Design review of the part built by this model. Coordinates are the model's own, in mm. Coordinates: 2 decimals unless noted, no trailing zeros. Loops run counter-clockwise (first coordinate to the right, second up) from the corner with the lowest first, then second, coordinate; pieces in that order, holes last. Notation, with made-up numbers: (80.5, 84.25) -> (100.5, 84.25) arc R30 ccw to (100.5, 116.25) -> close; hole circle Ø5 at (-21, 44). An arc over 180 degrees is marked (long way). Use one line per item in the form item = value. Start each with the question number.
1. Consider section A-A (z = -27.5). State the section outline as (x, y) points, then the cut area to 3 significant figures.
2. Consider section C-C (x = 1.1). State the section outline as (y, z) points.
3. Consider section B-B (y = -17). State the section outline as (x, z) points.
4. For pin 1 (5.5 mm diameter, centred on y = 17, z = 27.5, fed in from +X); pin 2 (3 mm diameter, centred on y = -17, z = 27.5, fed in from -X), all flat-tipped, find the tip position at first contact; note any pin that passes through.
5. Wall thickness on line 1 (Y direction, x = 2.7, z = 27.5); line 2 (Y direction, x = 0.45, z = -27.5); line 3 (Z direction, x = 2.25, y = 18): over which ranges is each line inside the solid? List them lowest first. Write a range as from..to.
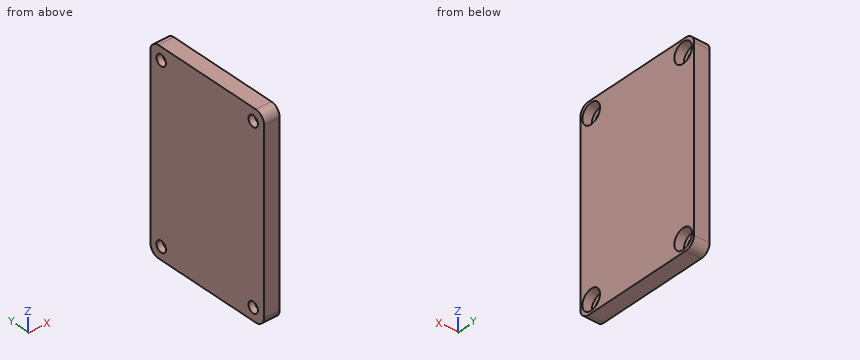
from build123d import *

# Parameters (mm, degrees)
BOSS_EXTRUDE1_DEPTH = 5
SKETCH2_R           = 1.75
CUT_EXTRUDE1_DEPTH  = 39.187039686
SKETCH3_R           = 3.25
CUT_EXTRUDE2_DEPTH  = 3


with BuildPart() as part:
    # Sketch1 → Boss-Extrude1 (new body)
    with BuildSketch(Plane.YZ):
        with BuildLine():
            Line((-18, -31.5), (18, -31.5))
            ThreePointArc((18, -31.5), (20.121320344, -30.621320344), (21, -28.5))
            Line((21, -28.5), (21, 28.5))
            ThreePointArc((21, 28.5), (20.121320344, 30.621320344), (18, 31.5))
            Line((18, 31.5), (-18, 31.5))
            ThreePointArc((-18, 31.5), (-20.121320344, 30.621320344), (-21, 28.5))
            Line((-21, 28.5), (-21, -28.5))
            ThreePointArc((-21, -28.5), (-20.121320344, -30.621320344), (-18, -31.5))
        make_face()
    extrude(amount=BOSS_EXTRUDE1_DEPTH)

    # Sketch2 → Cut-Extrude1 (cut, through all)
    with BuildSketch(Plane.YZ.offset(5)):
        with Locations(Location((-17, 27.5, 0), (0, 0, 270))):
            Circle(SKETCH2_R)
        with Locations(Location((17, 27.5, 0), (0, 0, 270))):
            Circle(SKETCH2_R)
        with Locations(Location((17, -27.5, 0), (0, 0, 270))):
            Circle(SKETCH2_R)
        with Locations(Location((-17, -27.5, 0), (0, 0, 270))):
            Circle(SKETCH2_R)
    extrude(amount=-CUT_EXTRUDE1_DEPTH, mode=Mode.SUBTRACT)

    # Sketch3 → Cut-Extrude2 (cut)
    with BuildSketch(Plane.YZ.offset(5)):
        with Locations(Location((17, 27.5, 0), (0, 0, 270))):
            Circle(SKETCH3_R)
        with Locations(Location((-17, 27.5, 0), (0, 0, 270))):
            Circle(SKETCH3_R)
        with Locations(Location((17, -27.5, 0), (0, 0, 270))):
            Circle(SKETCH3_R)
        with Locations(Location((-17, -27.5, 0), (0, 0, 270))):
            Circle(SKETCH3_R)
    extrude(amount=-CUT_EXTRUDE2_DEPTH, mode=Mode.SUBTRACT)


solid = part.part
Geometry check:
q1.outline = (0, -21) -> (5, -21) -> (5, -20.25) -> (2, -20.25) -> (2, -18.75) -> (0, -18.75) -> close; (0, -15.25) -> (2, -15.25) -> (2, -13.75) -> (5, -13.75) -> (5, 13.75) -> (2, 13.75) -> (2, 15.25) -> (0, 15.25) -> close; (0, 18.75) -> (2, 18.75) -> (2, 20.25) -> (5, 20.25) -> (5, 21) -> (0, 21) -> close
q1.area = 157 mm²
q2.outline = (-21, -28.5) arc R3 ccw to (-18, -31.5) -> (18, -31.5) arc R3 ccw to (21, -28.5) -> (21, 28.5) arc R3 ccw to (18, 31.5) -> (-18, 31.5) arc R3 ccw to (-21, 28.5) -> close; hole circle Ø3.5 at (-17, -27.5); hole circle Ø3.5 at (-17, 27.5); hole circle Ø3.5 at (17, -27.5); hole circle Ø3.5 at (17, 27.5)
q3.outline = (0, -31.5) -> (5, -31.5) -> (5, -30.75) -> (2, -30.75) -> (2, -29.25) -> (0, -29.25) -> close; (0, -25.75) -> (2, -25.75) -> (2, -24.25) -> (5, -24.25) -> (5, 24.25) -> (2, 24.25) -> (2, 25.75) -> (0, 25.75) -> close; (0, 29.25) -> (2, 29.25) -> (2, 30.75) -> (5, 30.75) -> (5, 31.5) -> (0, 31.5) -> close
q4.pin_1 = 2
q4.pin_2 = through
q5.line_1 = -21..-20.25, -13.75..13.75, 20.25..21
q5.line_2 = -21..-18.75, -15.25..15.25, 18.75..21
q5.line_3 = -31.5..-30.59, -24.41..24.41, 30.59..31.5
